from build123d import *

# Parameters (mm, degrees)
BOSS_EXTRUDE1_DEPTH = 30
SHELL1_START        = -645
SHELL1_OUTLINE_W    = 50
SHELL1_OUTLINE_H    = 40
SHELL1_DEPTH        = 1290
SHELL1_2_OUTLINE_W  = 50
SHELL1_2_OUTLINE_H  = 105
SHELL1_2_DEPTH      = 95
SHELL1_START_2      = 550
SHELL1_3_OUTLINE_W  = 50
SHELL1_3_OUTLINE_H  = 105
SHELL1_3_DEPTH      = 95
SKETCH2_R           = 5
CUT_EXTRUDE1_DEPTH  = 665.623953827
CUT_EXTRUDE2_REACH  = 666.624
SKETCH3_R           = 5


# Read off the part's stored shape, not the designer's step: Shell1
with BuildPart() as part:
    # Sketch1 → Boss-Extrude1 (new, symmetric)
    with BuildSketch(Plane.YZ):
        Polygon((-550, -25), (550, -25), (550, -125), (650, -125), (650, 25), (550, 25), (-550, 25), (-650, 25), (-650, -125), (-550, -125), align=None)
    extrude(amount=BOSS_EXTRUDE1_DEPTH, both=True)

    # Shell1 outline → Shell1 (cut)
    with BuildSketch(Plane(origin=(0, 0, 0), x_dir=(1, 0, 0), z_dir=(0, 1, 0)).offset(SHELL1_START)):
        Rectangle(SHELL1_OUTLINE_W, SHELL1_OUTLINE_H)
    extrude(amount=SHELL1_DEPTH, mode=Mode.SUBTRACT)

    # Shell1 2 outline → Shell1 2 (cut)
    with BuildSketch(Plane(origin=(0, 0, 0), x_dir=(1, 0, 0), z_dir=(0, 1, 0)).offset(SHELL1_START)):
        with Locations((0, 72.5)):
            Rectangle(SHELL1_2_OUTLINE_W, SHELL1_2_OUTLINE_H)
    extrude(amount=SHELL1_2_DEPTH, mode=Mode.SUBTRACT)

    # Shell1 3 outline → Shell1 3 (cut)
    with BuildSketch(Plane(origin=(0, 0, 0), x_dir=(1, 0, 0), z_dir=(0, 1, 0)).offset(SHELL1_START_2)):
        with Locations((0, 72.5)):
            Rectangle(SHELL1_3_OUTLINE_W, SHELL1_3_OUTLINE_H)
    extrude(amount=SHELL1_3_DEPTH, mode=Mode.SUBTRACT)

    # Sketch2 → Cut-Extrude1 (cut, through all)
    with BuildSketch(Plane.YZ.offset(30)):
        with Locations(Location((-575, -75, 0), (0, 0, 270))):
            Circle(SKETCH2_R)
        with Locations(Location((575, -75, 0), (0, 0, 270))):
            Circle(SKETCH2_R)
    extrude(amount=-CUT_EXTRUDE1_DEPTH, mode=Mode.SUBTRACT)

    # Sketch3 → Cut-Extrude2 (cut, up to next)
    with BuildSketch(Plane.YZ.offset(30), mode=Mode.PRIVATE) as cut_extrude2_sk1:
        with Locations(Location((-350, 15, 0), (0, 0, 270))):
            Circle(SKETCH3_R)
    cut_extrude2_tool1 = extrude(cut_extrude2_sk1.sketch, amount=-CUT_EXTRUDE2_REACH, mode=Mode.PRIVATE) & part.part
    # Sketch3 → Cut-Extrude2 (cut, up to next)
    with BuildSketch(Plane.YZ.offset(30), mode=Mode.PRIVATE) as cut_extrude2_sk2:
        with Locations(Location((-350, -15, 0), (0, 0, 270))):
            Circle(SKETCH3_R)
    cut_extrude2_tool2 = extrude(cut_extrude2_sk2.sketch, amount=-CUT_EXTRUDE2_REACH, mode=Mode.PRIVATE) & part.part
    # Sketch3 → Cut-Extrude2 (cut, up to next)
    with BuildSketch(Plane.YZ.offset(30), mode=Mode.PRIVATE) as cut_extrude2_sk3:
        with Locations(Location((-450, 15, 0), (0, 0, 90))):
            Circle(SKETCH3_R)
    cut_extrude2_tool3 = extrude(cut_extrude2_sk3.sketch, amount=-CUT_EXTRUDE2_REACH, mode=Mode.PRIVATE) & part.part
    # Sketch3 → Cut-Extrude2 (cut, up to next)
    with BuildSketch(Plane.YZ.offset(30), mode=Mode.PRIVATE) as cut_extrude2_sk4:
        with Locations(Location((-450, -15, 0), (0, 0, 270))):
            Circle(SKETCH3_R)
    cut_extrude2_tool4 = extrude(cut_extrude2_sk4.sketch, amount=-CUT_EXTRUDE2_REACH, mode=Mode.PRIVATE) & part.part
    # Sketch3 → Cut-Extrude2 (cut, up to next)
    with BuildSketch(Plane.YZ.offset(30), mode=Mode.PRIVATE) as cut_extrude2_sk5:
        with Locations(Location((450, -15, 0), (0, 0, 270))):
            Circle(SKETCH3_R)
    cut_extrude2_tool5 = extrude(cut_extrude2_sk5.sketch, amount=-CUT_EXTRUDE2_REACH, mode=Mode.PRIVATE) & part.part
    # Sketch3 → Cut-Extrude2 (cut, up to next)
    with BuildSketch(Plane.YZ.offset(30), mode=Mode.PRIVATE) as cut_extrude2_sk6:
        with Locations(Location((450, 15, 0), (0, 0, 270))):
            Circle(SKETCH3_R)
    cut_extrude2_tool6 = extrude(cut_extrude2_sk6.sketch, amount=-CUT_EXTRUDE2_REACH, mode=Mode.PRIVATE) & part.part
    # Sketch3 → Cut-Extrude2 (cut, up to next)
    with BuildSketch(Plane.YZ.offset(30), mode=Mode.PRIVATE) as cut_extrude2_sk7:
        with Locations(Location((350, -15, 0), (0, 0, 270))):
            Circle(SKETCH3_R)
    cut_extrude2_tool7 = extrude(cut_extrude2_sk7.sketch, amount=-CUT_EXTRUDE2_REACH, mode=Mode.PRIVATE) & part.part
    # Sketch3 → Cut-Extrude2 (cut, up to next)
    with BuildSketch(Plane.YZ.offset(30), mode=Mode.PRIVATE) as cut_extrude2_sk8:
        with Locations(Location((350, 15, 0), (0, 0, 90))):
            Circle(SKETCH3_R)
    cut_extrude2_tool8 = extrude(cut_extrude2_sk8.sketch, amount=-CUT_EXTRUDE2_REACH, mode=Mode.PRIVATE) & part.part
    add(cut_extrude2_tool1.solids().sort_by_distance((30, -350, 15))[0], mode=Mode.SUBTRACT)
    add(cut_extrude2_tool2.solids().sort_by_distance((30, -350, -15))[0], mode=Mode.SUBTRACT)
    add(cut_extrude2_tool3.solids().sort_by_distance((30, -450, 15))[0], mode=Mode.SUBTRACT)
    add(cut_extrude2_tool4.solids().sort_by_distance((30, -450, -15))[0], mode=Mode.SUBTRACT)
    add(cut_extrude2_tool5.solids().sort_by_distance((30, 450, -15))[0], mode=Mode.SUBTRACT)
    add(cut_extrude2_tool6.solids().sort_by_distance((30, 450, 15))[0], mode=Mode.SUBTRACT)
    add(cut_extrude2_tool7.solids().sort_by_distance((30, 350, -15))[0], mode=Mode.SUBTRACT)
    add(cut_extrude2_tool8.solids().sort_by_distance((30, 350, 15))[0], mode=Mode.SUBTRACT)


solid = part.part
Could you check a few things on this model? Use its own coordinates, in mm. A direction names the side the tool comes from. Give positions to 0.01 mm unless a question says otherwise; leave off trailing zeros. Loops run counter-clockwise (first coordinate to the right, second up) from the corner with the lowest first, then second, coordinate; pieces in that order, holes last. Notation, with made-up numbers: (15, 36.5) -> (42, 36.5) arc R17 cw to (42, 63.5) -> close; hole circle Ø2 at (39, 63.5). An arc over 180 degrees is marked (long way). Return JSON: item names as keys, results as strings.
Item 1: I'm going to push a flat-ended pin straight in: pin 1 (8 mm diameter, centred on y = 350, z = -15, fed in from +X). Where does the tip first touch, or does it pass through?
Geometry results:
{"pin 1": "stops at x = -25"}
Item 2: I need wall thicknesses on L1, parallel to Y at x = -28, z = -75; L2, parallel to Y at x = 28, z = 15; L3, parallel to Z at x = 28.8, y = -350. Which ranges of each line are inside material? Lowest first, please. Write a range as from..to.
Geometry results:
{"L1": "y = -650..-580, -570..-550, 550..570, 580..650", "L2": "y = -650..-455, -445..-355, -345..345, 355..445, 455..650", "L3": "z = -25..-20, -10..10, 20..25"}
Item 3: Which directions (+Z, -Z, +X, -X, +Y, -Y) give clear straight access to the entire face, cutting with the end or side of a thin tool? Please do faces 4 (the flat face through (-27, -608, -125)), 5 (the flat face through (-25, -9, -19)), 6 (the flat face through (0, -8, -25)), 7 (the flat face through (0, -645, -54)), 8 (the flat face through (-30, -9, -16)).
Geometry results:
{"face 4": "-Z, +X, -X, +Y, -Y", "face 5": "none", "face 6": "-Z, +X, -X", "face 7": "-Z", "face 8": "+Z, -Z, -X, +Y, -Y"}
Item 4: If we section it at C-C on z = -45.5: List the corners of the cut face in (x, y) for me.
Geometry results:
{"outline": "(-30, -650) -> (30, -650) -> (30, -550) -> (25, -550) -> (25, -645) -> (-25, -645) -> (-25, -550) -> (-30, -550) -> close; (-30, 550) -> (-25, 550) -> (-25, 645) -> (25, 645) -> (25, 550) -> (30, 550) -> (30, 650) -> (-30, 650) -> close"}
Item 5: If we section it at B-B on x = -4.5: List the corners of the cut face in (y, z) for me, plus the area to 4 significant figures.
Geometry results:
{"outline": "(-650, -125) -> (-645, -125) -> (-645, 20) -> (645, 20) -> (645, -125) -> (650, -125) -> (650, 25) -> (-650, 25) -> close; (-550, -25) -> (550, -25) -> (550, -20) -> (-550, -20) -> close", "area": "13,450 mm²"}
Item 6: We'd pull the mould along Y, two halves only. Please class faces 1 (the flat face through (0, -650, -49)), 2 (the flat face through (0, 9, 25)), 3 (the flat face through (0, -9, 20)): +Y half, -Y half, draft (parallel to the pull), parting line (faces both ways), or undercut.
Geometry results:
{"face 1": "-Y half", "face 2": "draft", "face 3": "undercut"}
Item 7: If we section it at A-A on y = 144: List the corners of the cut face in (x, z) for me, plus the area to 3 significant figures.
Geometry results:
{"outline": "(-30, -25) -> (30, -25) -> (30, 25) -> (-30, 25) -> close; hole (-25, -20) -> (25, -20) -> (25, 20) -> (-25, 20) -> close", "area": "1,000 mm²"}
